from build123d import *

# Parameters (mm, degrees)
ESQUISSE1_W        = 5
ESQUISSE1_H        = 5
BOSS_EXTRU_1_DEPTH = 5


with BuildPart() as part:
    # Esquisse1 → Boss.-Extru.1 (new body)
    with BuildSketch(Plane.XY):
        Polygon((-10, 188), (-22, 188), (-22, 154), (-34, 154), (-34, 149), (-32, 149), (-32, 150.5), (-27, 150.5), (-27, 149), (-22, 149), (-22, 139), (-27, 139), (-27, 137.5), (-32, 137.5), (-32, 139), (-34, 139), (-34, 134), (-22, 134), (-22, 54), (-34, 54), (-34, 49), (-32, 49), (-32, 50.5), (-27, 50.5), (-27, 49), (-22, 49), (-22, 39), (-27, 39), (-27, 37.5), (-32, 37.5), (-32, 39), (-34, 39), (-34, 34), (-22, 34), (-22, 0), (-10, 0), (-10, -12), (-5, -12), (-5, -10), (-6.5, -10), (-6.5, -5), (-5, -5), (-5, 0), (5, 0), (5, -5), (6.5, -5), (6.5, -10), (5, -10), (5, -12), (10, -12), (10, 0), (22, 0), (22, 34), (34, 34), (34, 39), (32, 39), (32, 37.5), (27, 37.5), (27, 39), (22, 39), (22, 49), (27, 49), (27, 50.5), (32, 50.5), (32, 49), (34, 49), (34, 54), (22, 54), (22, 134), (34, 134), (34, 139), (32, 139), (32, 137.5), (27, 137.5), (27, 139), (22, 139), (22, 149), (27, 149), (27, 150.5), (32, 150.5), (32, 149), (34, 149), (34, 154), (22, 154), (22, 188), (10, 188), (10, 200), (5, 200), (5, 198), (6.5, 198), (6.5, 193), (5, 193), (5, 188), (-5, 188), (-5, 193), (-6.5, 193), (-6.5, 198), (-5, 198), (-5, 200), (-10, 200), align=None)
        with Locations((-7.5, 48)):
            Rectangle(ESQUISSE1_W, ESQUISSE1_H, mode=Mode.SUBTRACT)
        with Locations((7.5, 48)):
            Rectangle(ESQUISSE1_W, ESQUISSE1_H, mode=Mode.SUBTRACT)
        with Locations((-7.5, 128)):
            Rectangle(ESQUISSE1_W, ESQUISSE1_H, mode=Mode.SUBTRACT)
        with Locations((7.5, 128)):
            Rectangle(ESQUISSE1_W, ESQUISSE1_H, mode=Mode.SUBTRACT)
    extrude(amount=BOSS_EXTRU_1_DEPTH)


solid = part.part
Source: CAD feature listing. Evaluate the final solid. Frame: model axes, mm. A direction names the side the tool comes from. Coordinates: 2 decimals unless noted, no trailing zeros. Loops run counter-clockwise (first coordinate to the right, second up) from the corner with the lowest first, then second, coordinate; pieces in that order, holes last. Notation, with made-up numbers: M 55.25,89 L 71.25,89 A30 cw 71.25,112 Z; hole C -39.75,-16 d8. An arc over 180 degrees is marked long. Answer in a Markdown table with one row per item.
Q1. Section A-A on x = 24. Return the cut outline in (y, z), plus the area to 3 significant figures.
Answers below:
| item | result |
|---|---|
| outline | M 34,0 L 39,0 L 39,5 L 34,5 Z; M 49,0 L 54,0 L 54,5 L 49,5 Z; M 134,0 L 139,0 L 139,5 L 134,5 Z; M 149,0 L 154,0 L 154,5 L 149,5 Z |
| area | 100 mm^2 |
Q2. Ray query, probe 1 along Y at (x, z) = (-24, 3.25); probe 2 along Y at (x, z) = (-9.5, 2.85); probe 3 along Y at (x, z) = (29, 2.45). Return the intervals inside material, ascending. Write a range as from..to.
Answers below:
| item | result |
|---|---|
| probe 1 | y = 34..39, 49..54, 134..139, 149..154 |
| probe 2 | y = -12..45.5, 50.5..125.5, 130.5..200 |
| probe 3 | y = 34..37.5, 50.5..54, 134..137.5, 150.5..154 |
Q3. First-contact query: pin 1 (1.5 mm diameter, centred on x = 16, z = 1.5, fed in from +Y); pin 2 (2.5 mm diameter, centred on x = -25, z = 2.5, fed in from -Y); pin 3 (2 mm diameter, centred on x = 33.5, z = 2, fed in from +Y); pin 4 (1.5 mm diameter, centred on x = -14.5, y = 14.5, fed in from -Z). Flat tips, straight axial feed; report the tip coordinate or a pass-through.
Answers below:
| item | result |
|---|---|
| pin 1 | stops at y = 188 |
| pin 2 | stops at y = 34 |
| pin 3 | stops at y = 154 |
| pin 4 | stops at z = 0 |
Q4. Draft query along X for faces 5 (the flat face through (0, 0, 2)), 6 (the flat face through (-22, 95, 2)), 7 (the flat face through (-16, 188, 2)). Return one class per face: pulls with the +X half, pulls with the -X half, needs draft (parallel to the pull), parting line crosses it, or undercut.
Answers below:
| item | result |
|---|---|
| face 5 | undercut |
| face 6 | pulls with the -X half |
| face 7 | needs draft |
Q5. Set-up query: faces 1 (the flat face through (-5, 48, 2)), 2 (the flat face through (22, 17, 2)), 3 (the flat face through (28, 54, 2)), 4 (the flat face through (-22, 171, 2)). Return all of +Z, -Z, +X, -X, +Y, -Y with unobstructed straight access to the full face (end or side cutting, diameter ignored); none if empty.
Answers below:
| item | result |
|---|---|
| face 1 | +Z, -Z |
| face 2 | +Z, -Z, +X, -Y |
| face 3 | +Z, -Z, +X |
| face 4 | +Z, -Z, -X, +Y |
Q6. Section B-B on z = 2.7. State how many separate pieces and enclosed holes the cut face has, plus the area to 3 significant figures.
Answers below:
| item | result |
|---|---|
| separate pieces | 1 |
| enclosed holes | 4 |
| area | 8,800 mm^2 |
Q7. Section C-C on y = 4. Return the cut outline in (x, z).
Answers below:
| item | result |
|---|---|
| outline | M -22,0 L 22,0 L 22,5 L -22,5 Z |
Q8. Section D-D on x = -12. Return the cut outline in (y, z), plus the area to 3 significant figures.
Answers below:
| item | result |
|---|---|
| outline | M 0,0 L 188,0 L 188,5 L 0,5 Z |
| area | 940 mm^2 |
